Geometry check sheet. Reference: the model listing, model coordinates, mm. A direction names the side the tool comes from. Round coordinates to 2 decimals unless told otherwise and drop trailing zeros. Write each loop counter-clockwise with the first axis right and the second up, starting at its lowest first coordinate (ties: lowest second). Pieces come first, ordered by that corner, then holes. Notation, with made-up numbers: (43, -30) -> (90, -30) arc R27 ccw to (90, -14) -> close; hole circle Ø5 at (51.5, 60.25). An arc over 180 degrees is marked (long way). One line per question, with ' | ' between items.
```python
from build123d import *


with BuildPart() as part:
    # Sketch1 → Revolve2 (revolve)
    with BuildSketch(Plane(origin=(0, 0, 0), x_dir=(0, 0, -1), z_dir=(1, 0, 0))):
        with BuildLine():
            Line((0, 145.188), (0, 165))
            Line((0, 165), (-7, 165))
            Line((-7, 165), (-10.388686575, 152.353249532))
            ThreePointArc((-10.388686575, 152.353249532), (-11.522683536, 150.656103145), (-13.455501073, 150))
            Line((-13.455501073, 150), (-300, 150))
            ThreePointArc((-300, 150), (-310.960991624, 149.173944589), (-321.674372861, 146.714439069))
            ThreePointArc((-321.674372861, 146.714439069), (-439.541828247, 109.825171624), (-557.228519945, 72.363221744))
            ThreePointArc((-557.228519945, 72.363221744), (-595.405893511, 44.780757498), (-610, 0))
            Line((-610, 0), (-608.984, 0))
            ThreePointArc((-608.984, 0), (-594.259282427, 44.625319466), (-555.868158289, 71.724360639))
            ThreePointArc((-555.868158289, 71.724360639), (-438.8556959, 107.09296389), (-321.674372861, 141.898020722))
            ThreePointArc((-321.674372861, 141.898020722), (-311.025475884, 144.220518359), (-300.154164534, 145))
            Line((-300.154164534, 145), (-10.388686575, 145))
            Line((-10.388686575, 145), (-7, 145.188))
            Line((-7, 145.188), (0, 145.188))
        make_face()
    revolve(axis=Axis((0, 0, 0), (0, 0, 1)))


solid = part.part
```
(1) Sectioned sample at A-A on z = 39.5. Record the cut outline in (x, y), then the cut area to 3 significant figures.
Resolved:
outline: circle Ø300 at (0, 0); hole circle Ø290 at (0, 0) | area: 4,630 mm2
(2) Material ranges on line 1 (X direction, y = 0, z = 195); line 2 (Y direction, x = 90, z = 358.5), recorded low to high.
Resolved:
line 1: x = -150 to -145, 145 to 150 | line 2: y = -100.97 to -95.23, 95.23 to 100.97
(3) Access from +Z, -Z, +X, -X, +Y, -Y to the whole of each face (thin tool, end or side, straight path). Record for faces 1 (the cylindrical face through (-43.554, 138.304, 153.243)), 2 (the cylindrical face through (-148.724, -19.527, 158.734)).
Resolved:
face 1: -Z | face 2: +Z
(4) Go/stop test with flat-tipped pins: pin 1 (1.5 mm diameter, centred on y = 69.5, z = 354.5, fed in from -X); pin 2 (8 mm diameter, centred on x = -50.5, z = 284.5, fed in from +Y); pin 3 (3 mm diameter, centred on x = 126, z = 83, fed in from +Y). Record where each tip stops, or that it passes through.
Resolved:
pin 1: stops at x = -118 | pin 2: stops at y = 142.61 | pin 3: stops at y = 83.66
(5) Draft check along Y on faces 3 (the cylindrical face through (141.735, -31.474, 3.451)), 4 (the cylindrical face through (161.076, -35.769, 3.549)), 5 (the flat face through (146, 1, 0)). Enter one of: +Y half, -Y half, draft (parallel to the pull), parting line (faces both ways), or undercut.
Resolved:
face 3: undercut | face 4: parting line | face 5: draft
